Could you check a few things on this model? Use its own coordinates, in mm. A direction names the side the tool comes from. Round coordinates to 2 decimals unless told otherwise and drop trailing zeros. Loops run counter-clockwise (first coordinate to the right, second up) from the corner with the lowest first, then second, coordinate; pieces in that order, holes last.
from build123d import *

# Parameters (mm, degrees)
SKETCH1_R           = 5.0535
SKETCH1_R_2         = 4.1047
BOSS_EXTRUDE1_DEPTH = 6.35
SKETCH1_3_R         = 4.1047
BOSS_EXTRUDE2_DEPTH = 11
FILLET2_R           = 0.5


with BuildPart() as part:
    # Sketch1 → Boss-Extrude1 (new body)
    with BuildSketch(Plane(origin=(0, 0, 0), x_dir=(1, 0, 0), z_dir=(0, 1, 0))):
        with Locations(Location((0, 0, 0), (0, 0, 270))):
            Circle(SKETCH1_R)
        Circle(SKETCH1_R_2, mode=Mode.SUBTRACT)
        Circle(SKETCH1_R_2)
    extrude(amount=BOSS_EXTRUDE1_DEPTH)

    # Sketch1_3 → Boss-Extrude2 (add)
    with BuildSketch(Plane(origin=(0, 0, 0), x_dir=(1, 0, 0), z_dir=(0, 1, 0))):
        with Locations(Location((0, 0, 0), (0, 0, 270))):
            Circle(SKETCH1_3_R)
    extrude(amount=-BOSS_EXTRUDE2_DEPTH)

    # Fillet2
    fillet2_edges = [part.edges().sort_by_distance(p)[0] for p in [
        (0, -11, -4.1047),
        (0, 0, -4.1047),
    ]]
    fillet(fillet2_edges, radius=FILLET2_R)


solid = part.part
Item 1: Will these pins go through, and if not, where does the flat tip stop? pin 1 (6 mm diameter, centred on y = -4, z = 4, fed in from +X); pin 2 (4 mm diameter, centred on y = 4.5, z = 3, fed in from -X).
Results list:
pin 1: stops at x = 3.98
pin 2: stops at x = -4.95
Item 2: If we section it at A-A, the plane z = 0: Please give me the cut outline in (x, y).
Results list:
outline: (-5.05, 0) - (-4.6, 0) arc R0.5 cw to (-4.1, -0.5) - (-4.1, -10.5) arc R0.5 ccw to (-3.6, -11) - (3.6, -11) arc R0.5 ccw to (4.1, -10.5) - (4.1, -0.5) arc R0.5 cw to (4.6, 0) - (5.05, 0) - (5.05, 6.35) - (-5.05, 6.35) - close
Item 3: If we section it at B-B, the plane x = 0: Please give me the cut outline in (y, z).
Results list:
outline: (-11, -3.6) arc R0.5 ccw to (-10.5, -4.1) - (-0.5, -4.1) arc R0.5 cw to (0, -4.6) - (0, -5.05) - (6.35, -5.05) - (6.35, 5.05) - (0, 5.05) - (0, 4.6) arc R0.5 cw to (-0.5, 4.1) - (-10.5, 4.1) arc R0.5 ccw to (-11, 3.6) - close
Item 4: If we section it at D-D, the plane y = -4.5: Please give me the cut outline in (x, z), then the cut area to 3 significant figures.
Results list:
outline: circle Ø8.21 at (0, 0)
area: 52.9 mm2
Item 5: For faces 1 (the flat face through (0, 6.35, 0)), 2 (the cylindrical face through (0.2, -5.4, -4.1)), which set-ups out of +Z, -Z, +X, -X, +Y, -Y let a thin tool reach every point of the face, with its end or its side?
Results list:
face 1: +Z, -Z, +X, -X, +Y
face 2: -Y
Item 6: If I drill on line 1 along Y through (x, z) = (-3.75, -3); line 2 along X through (y, z) = (1, -3.5); line 3 along Z through (x, y) = (1.5, 5.5), over which ranges is the centre line in solid material (lowest first)?
Results list:
line 1: y = 0 to 6.35
line 2: x = -3.65 to 3.65
line 3: z = -4.83 to 4.83
Item 7: If we section it at C-C, the plane y = 4.75: Please give me the cut outline in (x, z).
Results list:
outline: circle Ø10.11 at (0, 0)
